Input: part model. Units: mm. Frame: model coordinates. Face numbers are marked on the shaded views. A direction names the side the tool comes from. Coordinates: 2 decimals unless noted, no trailing zeros. Write each loop counter-clockwise with the first axis right and the second up, starting at its lowest first coordinate (ties: lowest second). Pieces come first, ordered by that corner, then holes. Notation, with made-up numbers: (21.25, 33.25) - (48.25, 33.25) arc R13 cw to (48.25, 42.25) - close; hole circle Ø9 at (-21, 68). An arc over 180 degrees is marked (long way). Put each result on its own line as item: value. Start each with the question number.
1. Access query for the marked faces 4, 5, 6, 7 and 8. Directions: +Z, -Z, +X, -X, +Y, -Y. A direction counts if a zero-diameter tool reaches every point of the face in a straight line with its end or side. Return the directions, or none.
2. Cut plane A-A, the plane x = 56.5. Return loops of the section in (y, z).
3. Cut plane C-C, the plane y = 38.5. Return loops of the section in (x, z), and give its area (3 significant figures).
4. Cut plane D-D, the plane x = 122. Return loops of the section in (y, z), and give its area (3 significant figures).
5. Pull-direction query (X, two-part tool) for the marked faces 1, 2 and 3; classes: released by +X, released by -X, zero draft, split by the parting line, or undercut.
6. Line query: line 1 (X direction, y = -12.5, z = 13.5); line 2 (Y direction, x = 129.5, z = 10.5); line 3 (Z direction, x = 26, y = 52.5). Output: solid intervals per line, ascending.
7. Cut plane B-B, the plane z = 4. Return loops of the section in (x, y), and give its area (3 significant figures).
8. Pin query (flat end, axial travel): pin 1 (12 mm diameter, centred on x = 47.5, y = 25.5, fed in from -Z); pin 2 (17 mm diameter, centred on y = -12.5, z = 24, fed in from +X); pin 3 (14 mm diameter, centred on x = 136, z = 7, fed in from -Y); pin 4 (5 mm diameter, centred on x = 61.5, y = -14, fed in from +Z). Return the tip coordinate at first contact, or that it passes through.
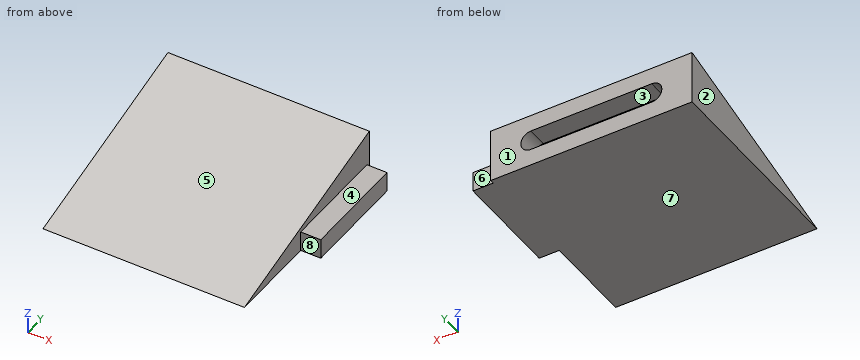
from build123d import *

# Parameters (mm, degrees)
F1_DEPTH = 127
F2_W     = 67.31
F2_H     = 12.7
F3_DEPTH = 12.7
F5_DEPTH = 12.7


with BuildPart() as f1:
    # F0 (on Right) → F1 (new body)
    with BuildSketch(Plane.YZ):
        Polygon((63.5, 34.029547), (-63.5, 0), (63.5, 0), align=None)
    extrude(amount=F1_DEPTH)

    # F2 (on face) → F3 (join)
    with BuildSketch(Plane.YZ.offset(127)):
        with Locations((27.305, 6.35)):
            Rectangle(F2_W, F2_H)
    extrude(amount=F3_DEPTH)

    # F4 (on face) → F5 (cut)
    with BuildSketch(Plane(origin=(0, 63.5, 0), x_dir=(-1, 0, 0), z_dir=(0, 1, 0))):
        with BuildLine():
            ThreePointArc((-101.6, 23.364774), (-107.95, 17.014774), (-101.6, 10.664774))
            Line((-101.6, 10.664774), (-25.4, 10.664774))
            ThreePointArc((-25.4, 10.664774), (-19.05, 17.014774), (-25.4, 23.364774))
            Line((-25.4, 23.364774), (-101.6, 23.364774))
        make_face()
    extrude(amount=-F5_DEPTH, mode=Mode.SUBTRACT)


solid = f1.part
Report:
1. face 4: +Z, +X, +Y, -Y
1. face 5: +Z, +X, -X, -Y
1. face 6: +Z, -Z, +X, +Y
1. face 7: -Z, +X, -X, +Y, -Y
1. face 8: +Z, -Z, +X, -Y
2. outline: (-63.5, 0) - (63.5, 0) - (63.5, 10.66) - (50.8, 10.66) - (50.8, 23.36) - (63.5, 23.36) - (63.5, 34.03) - close
3. outline: (0, 0) - (139.7, 0) - (139.7, 12.7) - (127, 12.7) - (127, 27.33) - (0, 27.33) - close
3. area: 3,630 mm^2
4. outline: (-63.5, 0) - (63.5, 0) - (63.5, 34.03) - close
4. area: 2,160 mm^2
5. face 1: zero draft
5. face 2: released by -X
5. face 3: undercut
6. line 1: x = 0 to 127
6. line 2: y = -6.35 to 60.96
6. line 3: z = 0 to 10.66, 23.36 to 31.08
7. outline: (0, -48.57) - (127, -48.57) - (127, -6.35) - (139.7, -6.35) - (139.7, 60.96) - (127, 60.96) - (127, 63.5) - (0, 63.5) - close
7. area: 15,100 mm^2
8. pin 1: stops at z = 0
8. pin 2: passes through
8. pin 3: stops at y = -6.35
8. pin 4: stops at z = 13.93
